Here's how the part is built. I have some questions about the finished solid (model axes, mm). Give positions to 0.01 mm unless a question says otherwise; leave off trailing zeros. Write each loop counter-clockwise with the first axis right and the second up, starting at its lowest first coordinate (ties: lowest second). Pieces come first, ordered by that corner, then holes. Notation, with made-up numbers: (69, -38) -> (121, -38) arc R25 ccw to (121, -7) -> close; hole circle Ø5 at (-23.75, 76). An arc over 180 degrees is marked (long way). Put each result on its own line as item: value. Start each with the question number.
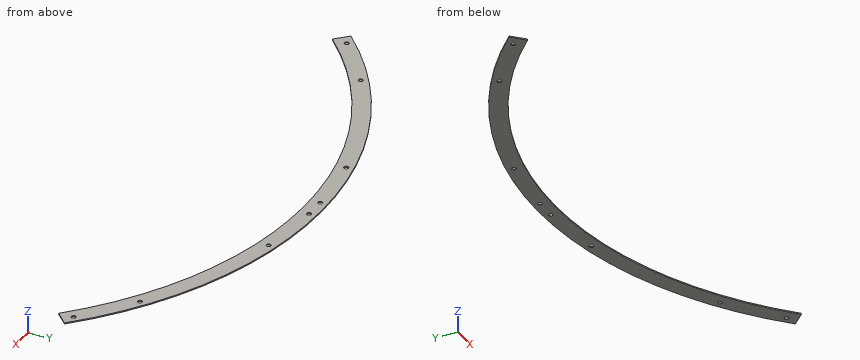
Autodesk Inventor part; units mm, degrees
ref_plane "YZ Plane" through (0, 0, 0) normal (1, 0, 0) x (0, 1, 0)
ref_plane "XZ Plane" through (0, 0, 0) normal (0, 1, 0) x (-1, 0, 0)
ref_plane "XY Plane" through (0, 0, 0) normal (0, 0, 1) x (1, 0, 0)
sketch "Sketch1" plane through (0, 0, 0) normal (0, 0, 1) x (1, 0, 0)
  circle A0 centre (0, 0) radius 650
  circle A1 centre (0, 0) radius 680
  line L0 (0, 0) -> (-480.8326, 480.8326)
  line L1 (0, 0) -> (0, 680)
  line L2 (0, 0) -> (480.8326, 480.8326)
  point P0 (-459.6194, 459.6194)
  point P1 (459.6194, 459.6194)
  dimension "d30" = 90
  dimension "d31" = 1360
  dimension "d32" = 1300
extrude "Plate1" add sketch "Sketch1" against normal blind 2 contours A0 L1 A1 L2 | L0 A1 L1 A0
sketch "Sketch2" plane through (0, 0, 0) normal (0, 0, 1) x (1, 0, 0)
  circle A0 centre (0, 0) radius 667.5
  arc A1 (480.8326, 480.8326) -> (-480.8326, 480.8326) centre (0, 0) ccw
  line L0 (0, 0) -> (480.8326, 480.8326) construction
  line L1 (0, 0) -> (458.5704, 485.0458) construction
  line L2 (370.8431, 555.006) -> (0, 0) construction
  line L3 (0, 0) -> (0, 667.5) construction
  line L4 (0, 0) -> (18.7209, 667.2374) construction
  line L5 (0, 0) -> (130.2228, 654.6742) construction
  line L6 (0, 0) -> (339.1403, 574.9262) construction
  line L7 (0, 0) -> (238.0449, 623.6112) construction
  dimension "d34" = 1335
  dimension "d35" = 1.607
  dimension "d36" = 9.643
  dimension "d44" = 1.607
  dimension "d45" = 9.643
  dimension "d49" = 3.214
  dimension "d50" = 9.643
hole "Hole1" at (458.5704, 485.0458, 0) at (370.8431, 555.006, 0) at (130.2228, 654.6742, 0) at (18.7209, 667.2374, 0) direction (0, 0, -1) diameter 8 end through all
pattern_circular "Circular Pattern1" count 2 over 45 about axis through (0, 0, -10) along (0, 0, 1) of "Hole1"
equation "\"d31\" = Колесо_диам_1"
equation "\"d32\" = Колесо_диам_2"
equation "\"d44\" = d35"
equation "\"d45\" = d36"
equation "\"d49\" = 2 * d35"
equation "\"d50\" = d36"
equation "\"d42\" = Thickness"
equation "\"d15\" = Thickness"
equation "\"BendRadius\" = Thickness"
equation "\"BendReliefWidth\" = Thickness"
equation "\"BendReliefDepth\" = 0.5 * Thickness"
equation "\"CornerReliefSize\" = 4 * Thickness"
equation "\"MinimumRemnant\" = 2 * Thickness"
equation "\"TransitionRadius\" = BendRadius"
equation "\"JacobiRadiusSize\" = BendRadius"
equation "\"GapSize\" = Thickness"
properties part number "DMF2.0 01 43 Gear rim 3"
1) I want a section at D-D, the plane x = 64.5. Write out the boundary of the cut face in (y, z).
2) I'm going to push flat-ended pins straight in: pin 1 Ø5 at (x, y) = (-458.57, 485.05) entering from -Z; pin 2 Ø10.5 at (x, y) = (18.72, 667.24) entering from +Z. Where does each tip first touch, or does it pass through?
3) I want a section at C-C, the plane y = 569.5. Write out the boundary of the cut face in (x, z).
4) I want a section at A-A, the plane y = 616. Write out the boundary of the cut face in (x, z).
5) I need wall thicknesses on probe 1 along X at (y, z) = (551.5, -1.9); probe 2 along X at (y, z) = (552, -0.75); probe 3 along X at (y, z) = (574, -1.4). Which ranges of each line are inside material? Lowest first, please.
6) I want a section at B-B, the plane z = -0.9. State how many separate pieces and enclosed holes the cut face has, and give its area (3 significant figures).
Established:
1. outline: (646.79, -2) -> (676.93, -2) -> (676.93, 0) -> (646.79, 0) -> close
2. pin 1: passes through
2. pin 2: stops at z = 0
3. outline: (-371.58, -2) -> (-313.32, -2) -> (-313.32, 0) -> (-371.58, 0) -> close; (313.32, -2) -> (371.58, -2) -> (371.58, 0) -> (313.32, 0) -> close
4. outline: (-288, -2) -> (-207.47, -2) -> (-207.47, 0) -> (-288, 0) -> close; (207.47, -2) -> (288, -2) -> (288, 0) -> (207.47, 0) -> close
5. probe 1: x = -397.8 to -372.77, -368.92 to -344.02, 344.02 to 368.92, 372.77 to 397.8
5. probe 2: x = -397.11 to -373.48, -368.2 to -343.21, 343.21 to 368.2, 373.48 to 397.11
5. probe 3: x = -364.59 to -305, 305 to 364.59
6. separate pieces: 1
6. enclosed holes: 8
6. area: 30,900 mm2
